Could you check a few things on this model? Use its own coordinates, in mm. A direction names the side the tool comes from. Give positions to 0.01 mm unless a question says otherwise; leave off trailing zeros. Order: outer loops, then holes, each group sorted by start corner. A loop starts at its lowest first (then second) coordinate and runs counter-clockwise, first axis right, second up. Notation, with made-up numbers: (45, 41.5) -> (94, 41.5) arc R22 cw to (94, 63.5) -> close; hole circle Ø5 at (37.25, -17). An arc over 180 degrees is marked (long way). One line per item, written item: value.
```python
from build123d import *

# Parameters (mm, degrees)
SKETCH1_R                        = 1.4732
BOSS_EXTRUDE1_DEPTH              = 2.9591
SKETCH4_W                        = 2.9591
SKETCH4_H                        = 6.35
CUT_EXTRUDE2_DEPTH               = 2.9591
BOSS_EXTRUDE5_DEPTH              = 2.9591
FILLET2_R                        = 1.27
FILLET3_R                        = 6.35
F_3_8_0_375_DIAMETER_HOLE1_D     = 9.525
F_3_8_0_375_DIAMETER_HOLE1_DEPTH = 6.35
F_3_8_0_375_DIAMETER_HOLE1_TIP   = 2.861598698
F_4_CLEARANCE_HOLE1_D            = 2.9464
F_4_CLEARANCE_HOLE1_DEPTH        = 6.35
F_4_CLEARANCE_HOLE1_TIP          = 0.885187864
F_4_CLEARANCE_HOLE2_D            = 2.9464
F_4_CLEARANCE_HOLE2_DEPTH        = 3.302
F_4_CLEARANCE_HOLE2_TIP          = 0.885187864
SKETCH23_W                       = 14.996716291
SKETCH23_H                       = 0.127
CUT_EXTRUDE4_DEPTH               = 2.9591


with BuildPart() as part:
    # Sketch1 → Boss-Extrude1 (new body)
    with BuildSketch(Plane.XY):
        with BuildLine():
            Line((6.35, -25.4), (6.35, -31.75))
            Line((6.35, -31.75), (-6.35, -31.75))
            Line((-6.35, -31.75), (-6.35, -25.4))
            Line((-6.35, -25.4), (-25.4, -25.4))
            Line((-25.4, -25.4), (-25.4, -6.35))
            Line((-25.4, -6.35), (-32.766, -6.35))
            ThreePointArc((-32.766, -6.35), (-39.116, 0), (-32.766, 6.35))
            Line((-32.766, 6.35), (-15.875, 6.35))
            Line((-15.875, 6.35), (-15.875, -12.7))
            Line((-15.875, -12.7), (-6.35, -12.7))
            Line((-6.35, -12.7), (-6.35, -9.7409))
            Line((-6.35, -9.7409), (6.35, -9.7409))
            Line((6.35, -9.7409), (6.35, -12.7))
            Line((6.35, -12.7), (15.875, -12.7))
            Line((15.875, -12.7), (15.875, 6.35))
            Line((15.875, 6.35), (32.766, 6.35))
            ThreePointArc((32.766, 6.35), (39.116, 0), (32.766, -6.35))
            Line((32.766, -6.35), (25.4, -6.35))
            Line((25.4, -6.35), (25.4, -25.4))
            Line((25.4, -25.4), (6.35, -25.4))
        make_face()
        with Locations((32.766, 0)):
            Circle(SKETCH1_R, mode=Mode.SUBTRACT)
        with Locations((-32.766, 0)):
            Circle(SKETCH1_R, mode=Mode.SUBTRACT)
        with BuildLine():
            Line((-5.08, -15.875), (5.08, -15.875))
            ThreePointArc((5.08, -15.875), (5.978025612, -16.246974388), (6.35, -17.145))
            Line((6.35, -17.145), (6.35, -20.955))
            ThreePointArc((6.35, -20.955), (5.978025612, -21.853025612), (5.08, -22.225))
            Line((5.08, -22.225), (-5.08, -22.225))
            ThreePointArc((-5.08, -22.225), (-5.978025612, -21.853025612), (-6.35, -20.955))
            Line((-6.35, -20.955), (-6.35, -17.145))
            ThreePointArc((-6.35, -17.145), (-5.978025612, -16.246974388), (-5.08, -15.875))
        make_face(mode=Mode.SUBTRACT)
    extrude(amount=BOSS_EXTRUDE1_DEPTH)

    # Sketch4 → Cut-Extrude2 (cut)
    with BuildSketch(Plane.XY.offset(2.9591)):
        with Locations((14.17955, -22.225)):
            Rectangle(SKETCH4_W, SKETCH4_H)
    cut_extrude2 = extrude(amount=-CUT_EXTRUDE2_DEPTH, mode=Mode.SUBTRACT)

    # Mirror2: Cut-Extrude2 across plane
    add(cut_extrude2.mirror(Plane(origin=(0, 0, 0), x_dir=(0, 0, 1), z_dir=(1, 0, 0))), mode=Mode.SUBTRACT)

    # Sketch10 → Boss-Extrude5 (add)
    with BuildSketch(Plane(origin=(0, 0, 0), x_dir=(-1, 0, 0), z_dir=(0, 0, -1))):
        Polygon((25.4, 6.35), (15.875, 6.35), (15.875, 0), (-15.875, 0), (-15.875, 6.35), (-25.4, 6.35), (-25.4, 15.875), (-9.525, 15.875), (-9.525, 81.541278797), (9.525, 81.541278797), (9.525, 15.875), (25.4, 15.875), align=None)
    extrude(amount=-BOSS_EXTRUDE5_DEPTH)

    # Fillet2
    fillet2_edges = [part.edges().sort_by_distance(p)[0] for p in [
        (15.875, 0, 1.47955),
        (-15.875, 0, 1.47955),
    ]]
    fillet(fillet2_edges, radius=FILLET2_R)

    # Fillet3
    fillet3_edges = [part.edges().sort_by_distance(p)[0] for p in [
        (-9.525, 15.875, 1.47955),
        (9.525, 15.875, 1.47955),
    ]]
    fillet(fillet3_edges, radius=FILLET3_R)

    # 3/8 (0.375) Diameter Hole1
    with Locations(Plane.XY.offset(2.9591)):
        with Locations((0, 68.841278797), (0, 18.041278797)):
            Hole(F_3_8_0_375_DIAMETER_HOLE1_D / 2, depth=F_3_8_0_375_DIAMETER_HOLE1_DEPTH)
            with Locations((0, 0, -(F_3_8_0_375_DIAMETER_HOLE1_DEPTH + F_3_8_0_375_DIAMETER_HOLE1_TIP / 2))):  # 118° drill point
                Cone(0, F_3_8_0_375_DIAMETER_HOLE1_D / 2, F_3_8_0_375_DIAMETER_HOLE1_TIP, mode=Mode.SUBTRACT)

    # #4 Clearance Hole1
    with Locations(Plane.XY.offset(2.9591)):
        with Locations((-5.858825791, 77.875104588), (-5.858825791, 43.441278797), (-5.858825791, 9.006498797), (5.858825791, 9.006498797), (5.858825791, 43.441278797), (5.858825791, 77.875104588)):
            Hole(F_4_CLEARANCE_HOLE1_D / 2, depth=F_4_CLEARANCE_HOLE1_DEPTH)
            with Locations((0, 0, -(F_4_CLEARANCE_HOLE1_DEPTH + F_4_CLEARANCE_HOLE1_TIP / 2))):  # 118° drill point
                Cone(0, F_4_CLEARANCE_HOLE1_D / 2, F_4_CLEARANCE_HOLE1_TIP, mode=Mode.SUBTRACT)

    # #4 Clearance Hole2
    with Locations(Plane.XY.offset(2.9591)):
        with Locations((-20.6375, 0), (20.6375, 0)):
            Hole(F_4_CLEARANCE_HOLE2_D / 2, depth=F_4_CLEARANCE_HOLE2_DEPTH)
            with Locations((0, 0, -(F_4_CLEARANCE_HOLE2_DEPTH + F_4_CLEARANCE_HOLE2_TIP / 2))):  # 118° drill point
                Cone(0, F_4_CLEARANCE_HOLE2_D / 2, F_4_CLEARANCE_HOLE2_TIP, mode=Mode.SUBTRACT)

    # Sketch23 → Cut-Extrude4 (cut)
    with BuildSketch(Plane.XY.offset(2.9591)):
        with Locations((-17.901641854, -25.3365)):
            Rectangle(SKETCH23_W, SKETCH23_H)
    cut_extrude4 = extrude(amount=-CUT_EXTRUDE4_DEPTH, mode=Mode.SUBTRACT)

    # Mirror3: Cut-Extrude4 across plane
    add(cut_extrude4.mirror(Plane(origin=(0, 0, 0), x_dir=(0, 0, 1), z_dir=(1, 0, 0))), mode=Mode.SUBTRACT)


solid = part.part
```
1) For faces 1 (the flat face through (29, 6.35, 1)), 2 (the flat face through (6.35, -11, 1)), 3 (the flat face through (21, -25.273, 2)), 4 (the flat face through (15.659, -22, 2)), which set-ups out of +Z, -Z, +X, -X, +Y, -Y let a thin tool reach every point of the face, with its end or its side?
Answer below:
face 1: +Z, -Z, +X, +Y
face 2: +Z, -Z
face 3: +Z, -Z, +X, -Y
face 4: +Z, -Z, -Y
2) If I drill on line 1 along X through (y, z) = (-8.5, 2.1) (3 decimals); line 2 along Y through (x, z) = (-7, 1.7); line 3 along Y through (x, z) = (33, 2.75), over which ranges is the centre line in solid material (lowest first)?
Answer below:
line 1: x = -25.4 to -15.875, 15.875 to 25.4
line 2: y = -25.4 to -12.7, 0 to 8.07, 9.94 to 42.51, 44.37 to 76.94, 78.81 to 81.54
line 3: y = -6.35 to -1.45, 1.45 to 6.35
3) Suppose I cut it at A-A, the plane x = 0. Write out the boundary of the cut face in (y, z) (3 decimals).
Answer below:
outline: (-31.75, 0) -> (-22.225, 0) -> (-22.225, 2.959) -> (-31.75, 2.959) -> close; (-15.875, 0) -> (-9.741, 0) -> (-9.741, 2.959) -> (-15.875, 2.959) -> close; (0, 0) -> (13.279, 0) -> (13.279, 2.959) -> (0, 2.959) -> close; (22.804, 0) -> (64.079, 0) -> (64.079, 2.959) -> (22.804, 2.959) -> close; (73.604, 0) -> (81.541, 0) -> (81.541, 2.959) -> (73.604, 2.959) -> close
4) Suppose I cut it at B-B, the plane x = -21. Write out the boundary of the cut face in (y, z) (3 decimals).
Answer below:
outline: (-25.273, 0) -> (-1.428, 0) -> (-1.428, 2.959) -> (-25.273, 2.959) -> close; (1.428, 0) -> (15.875, 0) -> (15.875, 2.959) -> (1.428, 2.959) -> close
5) For P1, Ø0.9, axis at y = -19, z = 2, coming from the +X side; P2, Ø1.5, axis at y = -12, z = 1.5, coming from the -X side; P3, Ø1.5, axis at x = -22.5, z = 1.5, coming from the +Y side (3 decimals), each with a flat end and sliding along its axis, tell me the tip position at first contact or that it passes through.
Answer below:
P1: stops at x = 25.4
P2: stops at x = -25.4
P3: stops at y = 15.875
6) We'd pull the mould along X, two halves only. Please class faces 5 (the cylindrical face through (-39.114, -0.14, 1.459)), 6 (the flat face through (-29, -6.35, 1)), 7 (the flat face through (0, -9.741, 1)), 8 (the flat face through (-12.7, -22, 2)): +X half, -X half, draft (parallel to the pull), parting line (faces both ways), or undercut.
Answer below:
face 5: -X half
face 6: draft
face 7: undercut
face 8: undercut
7) Suppose I cut it at D-D, the plane z = 0.75. State how many separate pieces and enclosed holes the cut face has, then the cut area to 3 significant figures.
Answer below:
separate pieces: 1
enclosed holes: 14
area: 3,060 mm2
8) Suppose I cut it at C-C, the plane x = 23.5. Write out the boundary of the cut face in (y, z) (3 decimals).
Answer below:
outline: (-25.273, 0) -> (15.875, 0) -> (15.875, 2.959) -> (-25.273, 2.959) -> close
